Part model, mm, in its own coordinate system. Face numbers are marked on the shaded views. A direction names the side the tool comes from. Give positions to 0.01 mm unless a question says otherwise; leave off trailing zeros. Order: outer loops, then holes, each group sorted by start corner. A loop starts at its lowest first (then second) coordinate and runs counter-clockwise, first axis right, second up. Notation, with made-up numbers: (-11, 73) - (0, 73) arc R32 ccw to (0, 112) - close; hole circle Ø8 at (57.5, 29). An arc over 180 degrees is marked (long way). One line per item, written item: value.
```python
from build123d import *

# Parameters (mm, degrees)
SKETCH_3_R                      = 2.8
CUT_EXTRUDE_2_DEPTH             = 4
SKETCH_8_R                      = 1.5
CUT_EXTRUDE_5_DEPTH             = 4
SKETCH_10_W                     = 24
SKETCH_10_H                     = 24
SKETCH_10_W_2                   = 20
SKETCH_10_H_2                   = 20
EXTRUDE_1_DEPTH                 = 15
EXTRUDE_2_DEPTH                 = 15
EXTRUDE_2_DEPTH_BACK            = 12
SKETCH_7_R                      = 5
SKETCH_7_R_2                    = 3.5
SKETCH_7_5_R                    = 3.5
CUT_EXTRUDE_6_DEPTH             = 12.360679775
FILLET_START                    = 6
FILLET_1_DEPTH                  = 15
FILLET_1_2_DEPTH                = 15
CUT_EXTRUDE_7_REACH             = 55.487
CUT_EXTRUDE_7_DIRECTION_2_DEPTH = 54.486637521


with BuildPart() as part:
    # 草图1 → 旋转1 (revolve)
    with BuildSketch(Plane.XY):
        with BuildLine():
            ThreePointArc((-15.620499352, 6), (-18.061145964, 3.183133409), (-20, 0))
            Line((-20, 0), (0, 0))
            Line((0, 0), (0, 6))
            Line((0, 6), (-15.620499352, 6))
        make_face()
    revolve(axis=Axis((0, 10, 0), (0, -1, 0)))

    # 草图3 → 切除-拉伸2 (cut)
    with BuildSketch(Plane.XZ):
        with Locations(Location((0, 0, 0), (0, 0, 270))):
            Circle(SKETCH_3_R)
    extrude(amount=-CUT_EXTRUDE_2_DEPTH, mode=Mode.SUBTRACT)

    # 草图8 → 切除-拉伸5 (cut)
    with BuildSketch(Plane.XZ.offset(-4)):
        with Locations(Location((0, 0, 0), (0, 0, 270))):
            Circle(SKETCH_8_R)
    extrude(amount=-CUT_EXTRUDE_5_DEPTH, mode=Mode.SUBTRACT)

    # 草图10 → 拉伸-薄壁1 (add)
    with BuildSketch(Plane(origin=(0, 6, 0), x_dir=(1, 0, 0), z_dir=(0, 1, 0))):
        Rectangle(SKETCH_10_W, SKETCH_10_H)
        Rectangle(SKETCH_10_W_2, SKETCH_10_H_2, mode=Mode.SUBTRACT)
    extrude(amount=EXTRUDE_1_DEPTH)

    # 草图7 → 凸台-拉伸2 (add, two sides: drawn at the far end of the back side and taken through both)
    with BuildSketch(Plane(origin=(22.360679775, 0, 0), x_dir=(0, 0, -1), z_dir=(1, 0, 0)).offset(-EXTRUDE_2_DEPTH_BACK)):
        with Locations((0, 13)):
            Circle(SKETCH_7_R)
        with Locations((0, 13)):
            Circle(SKETCH_7_R_2, mode=Mode.SUBTRACT)
    extrude(amount=EXTRUDE_2_DEPTH + EXTRUDE_2_DEPTH_BACK)

    # 草图7<5> → 切除-拉伸6 (cut)
    with BuildSketch(Plane(origin=(22.360679775, 0, 0), x_dir=(0, 0, -1), z_dir=(1, 0, 0))):
        with Locations((0, 13)):
            Circle(SKETCH_7_5_R)
    extrude(amount=-CUT_EXTRUDE_6_DEPTH, mode=Mode.SUBTRACT)

    # 圆角1: read off the stored shape, not the designer's step
    # 圆角1 outline → 圆角1 (cut)
    with BuildSketch(Plane(origin=(0, 0, 0), x_dir=(1, 0, 0), z_dir=(0, 1, 0)).offset(FILLET_START)):
        with BuildLine():
            ThreePointArc((-12, 7), (-10.535533906, 10.535533906), (-7, 12))
            Line((-7, 12), (-12, 12))
            Line((-12, 12), (-12, 7))
        make_face()
        with BuildLine():
            Line((12, 12), (7, 12))
            ThreePointArc((7, 12), (10.535533906, 10.535533906), (12, 7))
            Line((12, 7), (12, 12))
        make_face()
        with BuildLine():
            ThreePointArc((-7, -12), (-10.535533906, -10.535533906), (-12, -7))
            Line((-12, -7), (-12, -12))
            Line((-12, -12), (-7, -12))
        make_face()
        with BuildLine():
            Line((12, -12), (12, -7))
            ThreePointArc((12, -7), (10.535533906, -10.535533906), (7, -12))
            Line((7, -12), (12, -12))
        make_face()
    extrude(amount=FILLET_1_DEPTH, mode=Mode.SUBTRACT)

    # Fillet 1 2 outline → Fillet 1 2 (add)
    with BuildSketch(Plane(origin=(0, 0, 0), x_dir=(1, 0, 0), z_dir=(0, 1, 0)).offset(FILLET_START)):
        with BuildLine():
            Line((10, -10), (10, -5))
            ThreePointArc((10, -5), (8.535533906, -8.535533906), (5, -10))
            Line((5, -10), (10, -10))
        make_face()
        with BuildLine():
            ThreePointArc((5, 10), (8.535533906, 8.535533906), (10, 5))
            Line((10, 5), (10, 10))
            Line((10, 10), (5, 10))
        make_face()
        with BuildLine():
            Line((-10, -10), (-5, -10))
            ThreePointArc((-5, -10), (-8.535533906, -8.535533906), (-10, -5))
            Line((-10, -5), (-10, -10))
        make_face()
        with BuildLine():
            ThreePointArc((-10, 5), (-8.535533906, 8.535533906), (-5, 10))
            Line((-5, 10), (-10, 10))
            Line((-10, 10), (-10, 5))
        make_face()
    extrude(amount=FILLET_1_2_DEPTH)

    # 切除-拉伸7: up to this face of the body (flat: up to its plane)
    cut_extrude_7_end = Plane(part.part.faces().sort_by_distance((0, 13.5, -12))[0])
    # 草图13 → 切除-拉伸7 (cut, up to the picked face)
    with BuildSketch(Plane.XY.offset(12), mode=Mode.PRIVATE) as cut_extrude_7_sk1:
        with BuildLine():
            Line((-5, 17.5), (5, 17.5))
            ThreePointArc((5, 17.5), (6.5, 16), (5, 14.5))
            Line((5, 14.5), (-5, 14.5))
            ThreePointArc((-5, 14.5), (-6.5, 16), (-5, 17.5))
        make_face()
    cut_extrude_7_tool1 = split(extrude(cut_extrude_7_sk1.sketch, amount=-CUT_EXTRUDE_7_REACH, mode=Mode.PRIVATE), bisect_by=cut_extrude_7_end, keep=Keep.BOTH, mode=Mode.PRIVATE)
    # 草图13 → 切除-拉伸7 (cut, up to the picked face)
    with BuildSketch(Plane.XY.offset(12), mode=Mode.PRIVATE) as cut_extrude_7_sk2:
        with BuildLine():
            Line((-5, 12.5), (5, 12.5))
            ThreePointArc((5, 12.5), (6.5, 11), (5, 9.5))
            Line((5, 9.5), (-5, 9.5))
            ThreePointArc((-5, 9.5), (-6.5, 11), (-5, 12.5))
        make_face()
    cut_extrude_7_tool2 = split(extrude(cut_extrude_7_sk2.sketch, amount=-CUT_EXTRUDE_7_REACH, mode=Mode.PRIVATE), bisect_by=cut_extrude_7_end, keep=Keep.BOTH, mode=Mode.PRIVATE)
    add(cut_extrude_7_tool1.solids().sort_by(Axis((0, 16, 12), (0, 0, -1)))[0], mode=Mode.SUBTRACT)
    add(cut_extrude_7_tool2.solids().sort_by(Axis((0, 11, 12), (0, 0, -1)))[0], mode=Mode.SUBTRACT)

    # 草图13 → 切除-拉伸7 direction 2 (cut)
    with BuildSketch(Plane.XY.offset(12)):
        with BuildLine():
            Line((-5, 17.5), (5, 17.5))
            ThreePointArc((5, 17.5), (6.5, 16), (5, 14.5))
            Line((5, 14.5), (-5, 14.5))
            ThreePointArc((-5, 14.5), (-6.5, 16), (-5, 17.5))
        make_face()
        with BuildLine():
            Line((-5, 12.5), (5, 12.5))
            ThreePointArc((5, 12.5), (6.5, 11), (5, 9.5))
            Line((5, 9.5), (-5, 9.5))
            ThreePointArc((-5, 9.5), (-6.5, 11), (-5, 12.5))
        make_face()
    extrude(amount=CUT_EXTRUDE_7_DIRECTION_2_DEPTH, mode=Mode.SUBTRACT)


solid = part.part
```
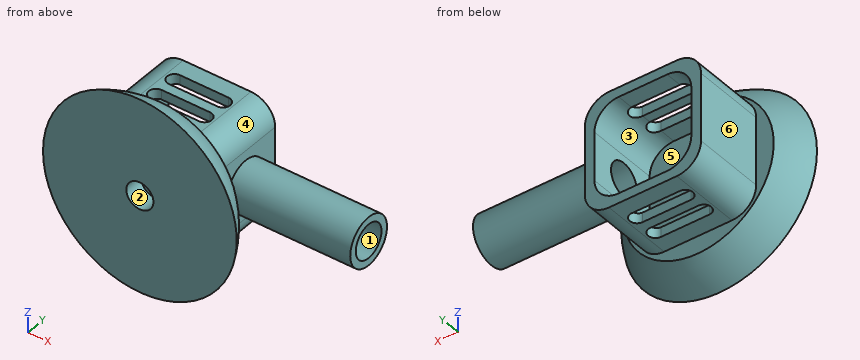
1) Which spindle directions (+Z, -Z, +X, -X, +Y, -Y) get a long thin tool onto all of the face, cutting with end or side? Do the marked faces 1, 2 and 3. Say none if no direction does.
Outcome:
face 1: +X
face 2: -Y
face 3: +Y
2) Cut at C-C, the plane x = 21.5. Give the cut face in (y, z), then the cut area to 3 significant figures.
Outcome:
outline: circle Ø10 at (13, 0); hole circle Ø7 at (13, 0)
area: 40.1 mm^2
3) Cut at D-D, the plane x = 13.5. Give the cut face in (y, z).
Outcome:
outline: (0, -14.76) arc R17.83 ccw to (6, -7.86) - (6, 7.86) arc R17.83 ccw to (0, 14.76) - close; circle Ø10 at (13, 0); hole circle Ø7 at (13, 0)
4) Drill centre lines: line 1 along X through (y, z) = (6.75, 2); line 2 along Y through (x, z) = (-6, -14); line 3 along X through (y, z) = (7.25, -8.5). Where is each one in solid material? Low to high. Write a range as from..to.
Outcome:
line 1: x = -12..-10, 10..12
line 2: y = 0..6
line 3: x = -11.77..-8.57, 8.57..11.77
5) Cut at A-A, the plane z = 0. Give the cut face in (x, y), then the cut area to 3 significant figures.
Outcome:
outline: (-20, 0) - (-2.8, 0) - (-2.8, 4) - (-1.5, 4) - (-1.5, 6) - (-10, 6) - (-10, 21) - (-12, 21) - (-12, 6) - (-15.62, 6) arc R22.36 ccw to start; (1.5, 4) - (2.8, 4) - (2.8, 0) - (20, 0) arc R22.36 ccw to (15.62, 6) - (12, 6) - (12, 8) - (37.36, 8) - (37.36, 9.5) - (10, 9.5) - (10, 6) - (1.5, 6) - close; (10, 16.5) - (37.36, 16.5) - (37.36, 18) - (12, 18) - (12, 21) - (10, 21) - close
area: 310 mm^2
6) Cut at B-B, the plane y = 19.5. Give the cut face in (x, z), then the cut area to 3 significant figures.
Outcome:
outline: (-12, -7) arc R5 ccw to (-7, -12) - (7, -12) arc R5 ccw to (12, -7) - (12, 7) arc R5 ccw to (7, 12) - (-7, 12) arc R5 ccw to (-12, 7) - close; hole (-10, -5) arc R5 ccw to (-5, -10) - (5, -10) arc R5 ccw to (10, -5) - (10, 5) arc R5 ccw to (5, 10) - (-5, 10) arc R5 ccw to (-10, 5) - close
area: 176 mm^2
7) Pin check, flat tips, straight feed: pin 1 (2 mm diameter, centred on y = 2.5, z = -1, fed in from -X); pin 2 (0.6 mm diameter, centred on x = -2.5, y = 13, fed in from +Z); pin 3 (3 mm diameter, centred on x = 30.5, y = 12, fed in from +Z). Stop position of each tip, or through.
Outcome:
pin 1: stops at x = -19.15
pin 2: stops at z = 12
pin 3: stops at z = 5
8) Mould opens along Z. For the marked faces 4, 5 and 6 say: released by +Z, released by -Z, zero draft, split by the parting line, or undercut.
Outcome:
face 4: released by +Z
face 5: undercut
face 6: zero draft
